from build123d import *

# Parameters (mm, degrees)
F1_DEPTH       = 6
F2_D           = 3
F3_D           = 1
F3_CBORE_D     = 1.5
F3_CBORE_DEPTH = 1


with BuildPart() as f1:
    # F0 (on Top) → F1 (new body)
    with BuildSketch(Plane.XY):
        with BuildLine():
            Line((52.7166165411, 30), (52.7166165411, 0))
            ThreePointArc((52.7166165411, 0), (67.7166165411, 15), (52.7166165411, 30))
        make_face()
        with BuildLine():
            Line((34.7231468186, 0), (52.7166165411, 0))
            ThreePointArc((52.7166165411, 0), (37.7166165411, 15), (52.7166165411, 30))
            Line((52.7166165411, 30), (35.3341475129, 30))
            Line((35.3341475129, 30), (-47.2833834589, 30))
            Line((-47.2833834589, 30), (-72.2833834589, 30))
            ThreePointArc((-72.2833834589, 30), (-75.8189173648, 28.5355339059), (-77.2833834589, 25))
            Line((-77.2833834589, 25), (-77.2833834589, 5))
            ThreePointArc((-77.2833834589, 5), (-75.8189173648, 1.4644660941), (-72.2833834589, 0))
            Line((-72.2833834589, 0), (16.729677096, 0))
            Line((16.729677096, 0), (34.7231468186, 0))
        make_face()
        with BuildLine():
            ThreePointArc((-69.7833834589, 19.5), (-68.9047038024, 21.6213203436), (-66.7833834589, 22.5))
            Line((-66.7833834589, 22.5), (-57.7833834589, 22.5))
            ThreePointArc((-57.7833834589, 22.5), (-55.6620631153, 21.6213203436), (-54.7833834589, 19.5))
            Line((-54.7833834589, 19.5), (-54.7833834589, 10.5))
            ThreePointArc((-54.7833834589, 10.5), (-55.6620631153, 8.3786796564), (-57.7833834589, 7.5))
            Line((-57.7833834589, 7.5), (-66.7833834589, 7.5))
            ThreePointArc((-66.7833834589, 7.5), (-68.9047038024, 8.3786796564), (-69.7833834589, 10.5))
            Line((-69.7833834589, 10.5), (-69.7833834589, 19.5))
        make_face(mode=Mode.SUBTRACT)
        with BuildLine():
            ThreePointArc((52.7166165411, 30), (37.7166165411, 15), (52.7166165411, 0))
            Line((52.7166165411, 0), (52.7166165411, 30))
        make_face()
    extrude(amount=F1_DEPTH)

    # F2 (through all)
    with Locations(Plane(origin=(0, 0, 0), x_dir=(1, 0, 0), z_dir=(0, 0, -1))):
        with Locations((52.7166165411, -15)):
            Hole(F2_D / 2)

    # F3 (through all)
    with Locations(Plane(origin=(0, 0, 0), x_dir=(1, 0, 0), z_dir=(0, 0, -1))):
        with Locations((55.7166165411, -18), (55.7166165411, -12), (49.7166165411, -12), (49.7166165411, -18)):
            CounterBoreHole(F3_D / 2, F3_CBORE_D / 2, F3_CBORE_DEPTH)


solid = f1.part
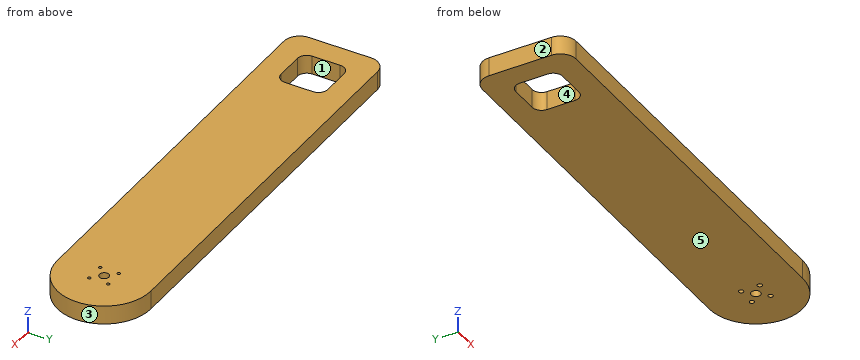
Work out the finished part from the listing and answer in its coordinate system (mm). Face numbers are marked on the shaded views. A direction names the side the tool comes from. Give positions to 0.01 mm unless a question says otherwise; leave off trailing zeros. Order: outer loops, then holes, each group sorted by start corner. A loop starts at its lowest first (then second) coordinate and runs counter-clockwise, first axis right, second up. Notation, with made-up numbers: (41, -3.5) -> (60, -3.5) arc R17 cw to (60, 15.5) -> close; hole circle Ø5 at (1.5, 17.25). An arc over 180 degrees is marked (long way). Answer as a JSON object with one key per item and string values. Group by question number.
1. Section B-B on y = 15 is taken. Determine the outline of the cut face in (x, z), plus the area to 3 significant figures.
2. Consider line 1 along X through (y, z) = (15, 3.55); line 2 along X through (y, z) = (12, 0.35); line 3 along Y through (x, z) = (-65, 0.75). Determine where each line is inside the solid, lowest interval first. Write a range as [from, to].
3. A tool of negligible diameter and unlimited length cuts with its end or side. For the marked faces 1 and 2, from which of +Z, -Z, +X, -X, +Y, -Y can it reach the whole face along a straight path? Write none if from no direction.
4. The mould has two halves that part along X. Classify the marked faces 3, 4 and 5: released by +X, released by -X, zero draft, split by the parting line, or undercut.
5. Section C-C on y = 2.75 is taken. Determine the outline of the cut face in (x, z), plus the area to 3 significant figures.
6. Section A-A on x = -61.5 is taken. Determine the outline of the cut face in (y, z).
7. A flat-ended cylindrical pin translates along its axis: pin 1 Ø1.2 at (x, y) = (49.72, 18) entering from -Z. Find the tip coordinate at first contact, or state that the pin passes through.
Result sheet:
{
 "1": {"outline": "(-77.28, 0) -> (-69.78, 0) -> (-69.78, 6) -> (-77.28, 6) -> close; (-54.78, 0) -> (51.22, 0) -> (51.22, 6) -> (-54.78, 6) -> close; (54.22, 0) -> (67.72, 0) -> (67.72, 6) -> (54.22, 6) -> close", "area": "762 mm^2"},
 "2": {"line 1": "x = [-77.28, -69.78], [-54.78, 51.22], [54.22, 67.72]", "line 2": "x = [-77.28, -69.78], [-54.78, 48.97], [50.47, 54.97], [56.47, 67.41]", "line 3": "y = [0, 7.5], [22.5, 30]"},
 "3": {"face 1": "+Z, -Z", "face 2": "+Z, -Z, -X, +Y, -Y"},
 "4": {"face 3": "released by +X", "face 4": "undercut", "face 5": "zero draft"},
 "5": {"outline": "(-76.75, 0) -> (61.37, 0) -> (61.37, 6) -> (-76.75, 6) -> close", "area": "829 mm^2"},
 "6": {"outline": "(0, 0) -> (7.5, 0) -> (7.5, 6) -> (0, 6) -> close; (22.5, 0) -> (30, 0) -> (30, 6) -> (22.5, 6) -> close"},
 "7": {"pin 1": "stops at z = 1"}
}
